```python
from build123d import *

# Parameters (mm, degrees)
BOSS_EXTRUDE1_DEPTH = 3.175
CUT_EXTRUDE1_DEPTH  = 4.175


with BuildPart() as part:
    # Sketch1 → Boss-Extrude1 (new body)
    with BuildSketch(Plane.XY):
        Polygon((0, 0), (50.8, 0), (50.8, -82.55), (0, -82.55), (0, -88.9), (44.721203233, -88.9), (44.721203233, -152.4), (9.928151849, -152.4), (9.928151849, -158.75), (61.345154174, -158.75), (66.833453826, -141.575386567), (66.833453826, -57.719185396), (58.42, 6.35), (0, 6.35), align=None)
    extrude(amount=BOSS_EXTRUDE1_DEPTH)

    # Sketch2 → Cut-Extrude1 (cut, through all)
    with BuildSketch(Plane.XY.offset(3.175)):
        with BuildLine():
            Line((4.696138357, 4.936538246), (14.893802938, 4.936538246))
            ThreePointArc((14.893802938, 4.936538246), (16.462065142, 3.368276042), (14.893802938, 1.800013839))
            Line((14.893802938, 1.800013839), (4.696138357, 1.800013839))
            ThreePointArc((4.696138357, 1.800013839), (3.127876153, 3.368276042), (4.696138357, 4.936538246))
        make_face()
        with BuildLine():
            Line((4.696138357, -83.929673164), (14.893802938, -83.929673164))
            ThreePointArc((14.893802938, -83.929673164), (16.462065142, -85.497935368), (14.893802938, -87.066197572))
            Line((14.893802938, -87.066197572), (4.696138357, -87.066197572))
            ThreePointArc((4.696138357, -87.066197572), (3.127876153, -85.497935368), (4.696138357, -83.929673164))
        make_face()
    extrude(amount=-CUT_EXTRUDE1_DEPTH, mode=Mode.SUBTRACT)


solid = part.part
```
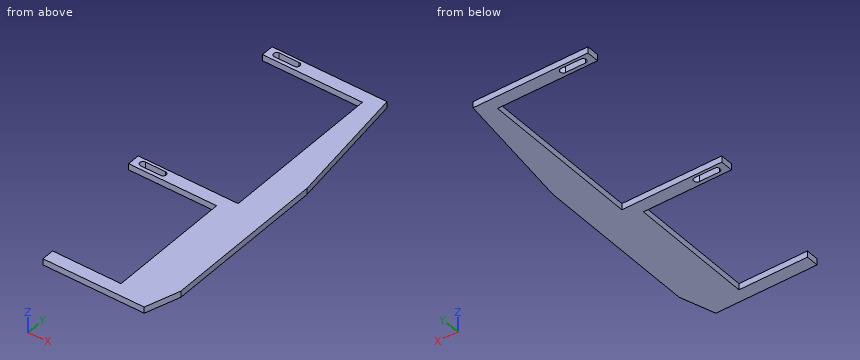
Input: part model. Units: mm. Frame: model coordinates. Coordinates: 2 decimals unless noted, no trailing zeros. Loops run counter-clockwise (first coordinate to the right, second up) from the corner with the lowest first, then second, coordinate; pieces in that order, holes last. Notation, with made-up numbers: M 27.25,-21.5 L 74.25,-21.5 A17 ccw 74.25,8.5 Z; hole C 34.25,10 d3. An arc over 180 degrees is marked long. One line per item, written item: value.
(1) Section D-D (z = 1.4). Output: boundary loops of the cut face in (x, y).
Filled in:
outline: M 0,-88.9 L 44.72,-88.9 L 44.72,-152.4 L 9.93,-152.4 L 9.93,-158.75 L 61.35,-158.75 L 66.83,-141.58 L 66.83,-57.72 L 58.42,6.35 L 0,6.35 L 0,0 L 50.8,0 L 50.8,-82.55 L 0,-82.55 Z; hole M 4.7,-87.07 L 14.89,-87.07 A1.57 ccw 14.89,-83.93 L 4.7,-83.93 A1.57 ccw Z; hole M 4.7,1.8 L 14.89,1.8 A1.57 ccw 14.89,4.94 L 4.7,4.94 A1.57 ccw Z
(2) Pin query (flat end, axial travel): pin 1 (1.6 mm diameter, centred on y = -155.5, z = 1, fed in from -X); pin 2 (1.6 mm diameter, centred on y = -33.5, z = 2, fed in from -X). Return the tip coordinate at first contact, or that it passes through.
Filled in:
pin 1: x = 9.93
pin 2: x = 50.8
(3) Section B-B (y = -85.5). Output: boundary loops of the cut face in (x, z) (3 decimals).
Filled in:
outline: M 0,0 L 3.128,0 L 3.128,3.175 L 0,3.175 Z; M 16.462,0 L 66.833,0 L 66.833,3.175 L 16.462,3.175 Z
(4) Line query: line 1 along Y through (x, z) = (25, 2.7); line 2 along Y through (x, z) = (10, 0.55); line 3 along X through (y, z) = (-85.5, 0.85). Output: solid intervals per line, ascending. Write a range as from..to.
Filled in:
line 1: -158.75..-152.4, -88.9..-82.55, 0..6.35
line 2: -158.75..-152.4, -88.9..-87.07, -83.93..-82.55, 0..1.8, 4.94..6.35
line 3: 0..3.13, 16.46..66.83
(5) Section C-C (x = 6.5). Output: boundary loops of the cut face in (y, z) (3 decimals).
Filled in:
outline: M -88.9,0 L -87.066,0 L -87.066,3.175 L -88.9,3.175 Z; M -83.93,0 L -82.55,0 L -82.55,3.175 L -83.93,3.175 Z; M 0,0 L 1.8,0 L 1.8,3.175 L 0,3.175 Z; M 4.937,0 L 6.35,0 L 6.35,3.175 L 4.937,3.175 Z
(6) Section A-A (x = 25). Output: boundary loops of the cut face in (y, z) (3 decimals), and give its area (3 significant figures).
Filled in:
outline: M -158.75,0 L -152.4,0 L -152.4,3.175 L -158.75,3.175 Z; M -88.9,0 L -82.55,0 L -82.55,3.175 L -88.9,3.175 Z; M 0,0 L 6.35,0 L 6.35,3.175 L 0,3.175 Z
area: 60.5 mm^2
